Could you check a few things on this model? Use its own coordinates, in mm. A direction names the side the tool comes from. Give positions to 0.01 mm unless a question says otherwise; leave off trailing zeros. Order: outer loops, then holes, each group sorted by start corner. A loop starts at its lowest first (then second) coordinate and runs counter-clockwise, first axis right, second up. Notation, with made-up numbers: M 5.25,-17.5 L 24.25,-17.5 A28 ccw 24.25,10.5 Z; hole C 15,81 d7. An arc over 180 degrees is marked long. Answer in a Markdown table with one row per item. Add a question column.
```python
from build123d import *

# Parameters (mm, degrees)
SKETCH1_W           = 21.59
SKETCH1_H           = 5.334
BOSS_EXTRUDE1_DEPTH = 5.334
SKETCH2_R           = 6
CUT_EXTRUDE1_DEPTH  = 5.334


with BuildPart() as part:
    # Sketch1 → Boss-Extrude1 (new body)
    with BuildSketch(Plane.XY):
        Polygon((-36.2, 24.449992223), (-23.5, 24.449992223), (-23.5, 42.483992223), (23.49, 42.483992223), (23.49, 24.449992223), (36.2, 24.449992223), (36.2, -7.777e-06), (18.1, -26.619054692), (-18.1, -26.619054692), (-36.2, 2.462571049), align=None)
        with Locations((-0.005, 32.451)):
            Rectangle(SKETCH1_W, SKETCH1_H, mode=Mode.SUBTRACT)
    extrude(amount=BOSS_EXTRUDE1_DEPTH)

    # Sketch2 → Cut-Extrude1 (cut)
    with BuildSketch(Plane.XY.offset(5.334)):
        with Locations((0, -7.112000122)):
            Circle(SKETCH2_R)
    extrude(amount=-CUT_EXTRUDE1_DEPTH, mode=Mode.SUBTRACT)


solid = part.part
```
1. Suppose I cut it at B-B on z = 2.9. List the corners of the cut face in (x, y) for me, plus the area to 3 significant figures.
2. Will these pins go through, and if not, where does the flat tip stop? P1, Ø15.5, axis at x = 0, y = -7.112, coming from the +Z side; P2, Ø2.5, axis at y = 30.5, z = 4, coming from the +X side; P3, Ø1.6, axis at x = 33, z = 3, coming from the +Y side; P4, Ø2, axis at y = -19, z = 1, coming from the +X side.
3. Suppose I cut it at D-D on y = -19. List the corners of the cut face in (x, z) for me, plus the area to 3 significant figures.
4. Suppose I cut it at C-C on x = -19. List the corners of the cut face in (y, z) for me, plus the area to 3 significant figures.
5. Thinking about a two-plate mould opening in X: for faces 1 (the cylindrical face through (-4.422, -3.057, 2.704)), 2 (the flat face through (27.28, -13.12, 2.63)), 3 (the flat face through (-36.2, 13, 3)), 4 (the flat face through (1, 8, 0)), which applies, pulls with the +X half, pulls with the -X half, needs draft (parallel to the pull), parting line crosses it, or undercut?
6. For faces 5 (the flat face through (36.2, 12, 3)), 6 (the flat face through (0, 42.484, 3)), 7 (the flat face through (-23.5, 33, 3)), 8 (the flat face through (0, 35.118, 3)), 9 (the flat face through (30, 24.45, 3)), which set-ups out of +Z, -Z, +X, -X, +Y, -Y let a thin tool reach every point of the face, with its end or its side?
7. If I drill on line 1 along Y through (x, z) = (0, 2.3); line 2 along Y through (x, z) = (-5, 5.1); line 3 along X through (y, z) = (32.5, 0.85), over which ranges is the centre line in solid material (lowest first)? Write a range as [from, to].
8. Suppose I cut it at A-A on x = 0. List the corners of the cut face in (y, z) for me, plus the area to 3 significant figures.
Findings below:
| question | item | result |
|---|---|---|
| 1 | outline | M -36.2,2.46 L -18.1,-26.62 L 18.1,-26.62 L 36.2,0 L 36.2,24.45 L 23.49,24.45 L 23.49,42.48 L -23.5,42.48 L -23.5,24.45 L -36.2,24.45 Z; hole M -10.8,29.78 L 10.79,29.78 L 10.79,35.12 L -10.8,35.12 Z; hole C 0,-7.11 d12 |
| 1 | area | 3,810 mm2 |
| 2 | P1 | z = 5.33 |
| 2 | P2 | x = 23.49 |
| 2 | P3 | y = 24.45 |
| 2 | P4 | x = 23.96 |
| 3 | outline | M -22.84,0 L 23.28,0 L 23.28,5.33 L -22.84,5.33 Z |
| 3 | area | 246 mm2 |
| 4 | outline | M -25.17,0 L 42.48,0 L 42.48,5.33 L -25.17,5.33 Z |
| 4 | area | 361 mm2 |
| 5 | face 1 | undercut |
| 5 | face 2 | pulls with the +X half |
| 5 | face 3 | pulls with the -X half |
| 5 | face 4 | needs draft |
| 6 | face 5 | +Z, -Z, +X, +Y, -Y |
| 6 | face 6 | +Z, -Z, +X, -X, +Y |
| 6 | face 7 | +Z, -Z, -X, +Y |
| 6 | face 8 | +Z, -Z |
| 6 | face 9 | +Z, -Z, +X, +Y |
| 7 | line 1 | [-26.62, -13.11], [-1.11, 29.78], [35.12, 42.48] |
| 7 | line 2 | [-26.62, -10.43], [-3.8, 29.78], [35.12, 42.48] |
| 7 | line 3 | [-23.5, -10.8], [10.79, 23.49] |
| 8 | outline | M -26.62,0 L -13.11,0 L -13.11,5.33 L -26.62,5.33 Z; M -1.11,0 L 29.78,0 L 29.78,5.33 L -1.11,5.33 Z; M 35.12,0 L 42.48,0 L 42.48,5.33 L 35.12,5.33 Z |
| 8 | area | 276 mm2 |
